Check sheet for the drawn part. Datum: minimum x, y, z corner. Units: mm. A direction names the side the tool comes from. Coordinates: 2 decimals unless noted, no trailing zeros. Order: outer loops, then holes, each group sorted by start corner. A loop starts at its lowest first (then second) coordinate and runs counter-clockwise, first axis right, second up.
Q1. Draft check along Z on the marked faces 1, 2 and 3. Enter one of: pulls with the +Z half, pulls with the -Z half, needs draft (parallel to the pull), parting line crosses it, or undercut.
Q2. Set-up check for the marked faces 4 and 5: record each of +Z, -Z, +X, -X, +Y, -Y from which the full face is reachable in a straight line by a thin tool's end or side.
Q3. Depth check by flat-ended pin: P1, Ø1.6, axis at y = 3, z = 5.5, coming from the +X side. Enter the tip coordinate at first touch or a pass-through.
Q4. Cross-section at D-D, the plane y = 2.35. Record the boundary of the cut face in (x, z), and give its area (3 significant figures).
Q5. Cross-section at C-C, the plane x = 0.75. Record the boundary of the cut face in (y, z).
Q6. Thickness scan on line 1 (Z direction, x = 5, y = 4.3); line 2 (Z direction, x = 3.3, y = 3); line 3 (Y direction, x = 1.7, z = 5.5). Record the ranges inside material, lowest first.
Q7. Cross-section at B-B, the plane x = 3. Record the boundary of the cut face in (y, z).
Q8. Cross-section at A-A, the plane y = 3. Record the boundary of the cut face in (x, z).
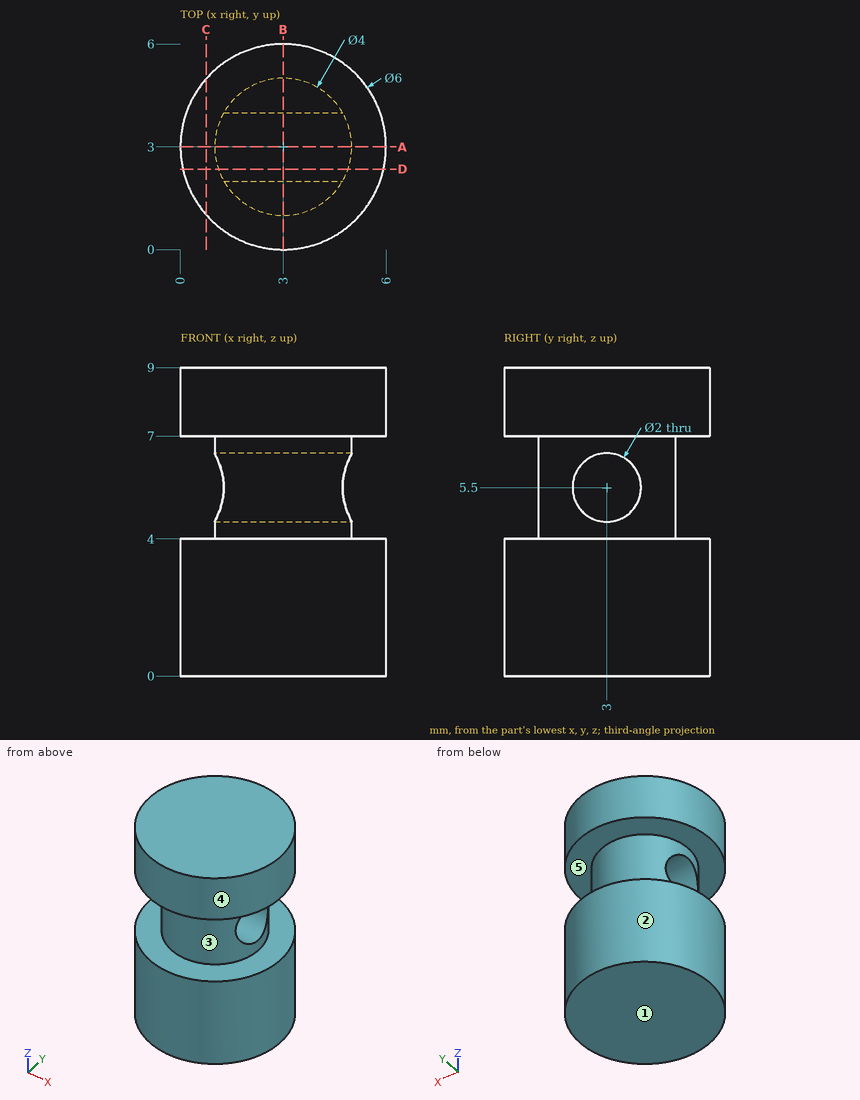
Check values:
1. face 1: pulls with the -Z half
1. face 2: needs draft
1. face 3: undercut
2. face 4: +Z, -Z
2. face 5: none
3. P1: passes through
4. outline: (0.07, 0) - (5.93, 0) - (5.93, 4) - (4.89, 4) - (4.89, 4.74) - (1.11, 4.74) - (1.11, 4) - (0.07, 4) - close; (0.07, 7) - (1.11, 7) - (1.11, 6.26) - (4.89, 6.26) - (4.89, 7) - (5.93, 7) - (5.93, 9) - (0.07, 9) - close
4. area: 40.7 mm2
5. outline: (1.02, 0) - (4.98, 0) - (4.98, 4) - (1.02, 4) - close; (1.02, 7) - (4.98, 7) - (4.98, 9) - (1.02, 9) - close
6. line 1: z = 0 to 4, 7 to 9
6. line 2: z = 0 to 4.5, 6.5 to 9
6. line 3: y = 1.48 to 2, 4 to 4.52
7. outline: (0, 0) - (6, 0) - (6, 4) - (5, 4) - (5, 7) - (6, 7) - (6, 9) - (0, 9) - (0, 7) - (1, 7) - (1, 4) - (0, 4) - close; hole circle Ø2 at (3, 5.5)
8. outline: (0, 0) - (6, 0) - (6, 4) - (5, 4) - (5, 4.5) - (1, 4.5) - (1, 4) - (0, 4) - close; (0, 7) - (1, 7) - (1, 6.5) - (5, 6.5) - (5, 7) - (6, 7) - (6, 9) - (0, 9) - close
